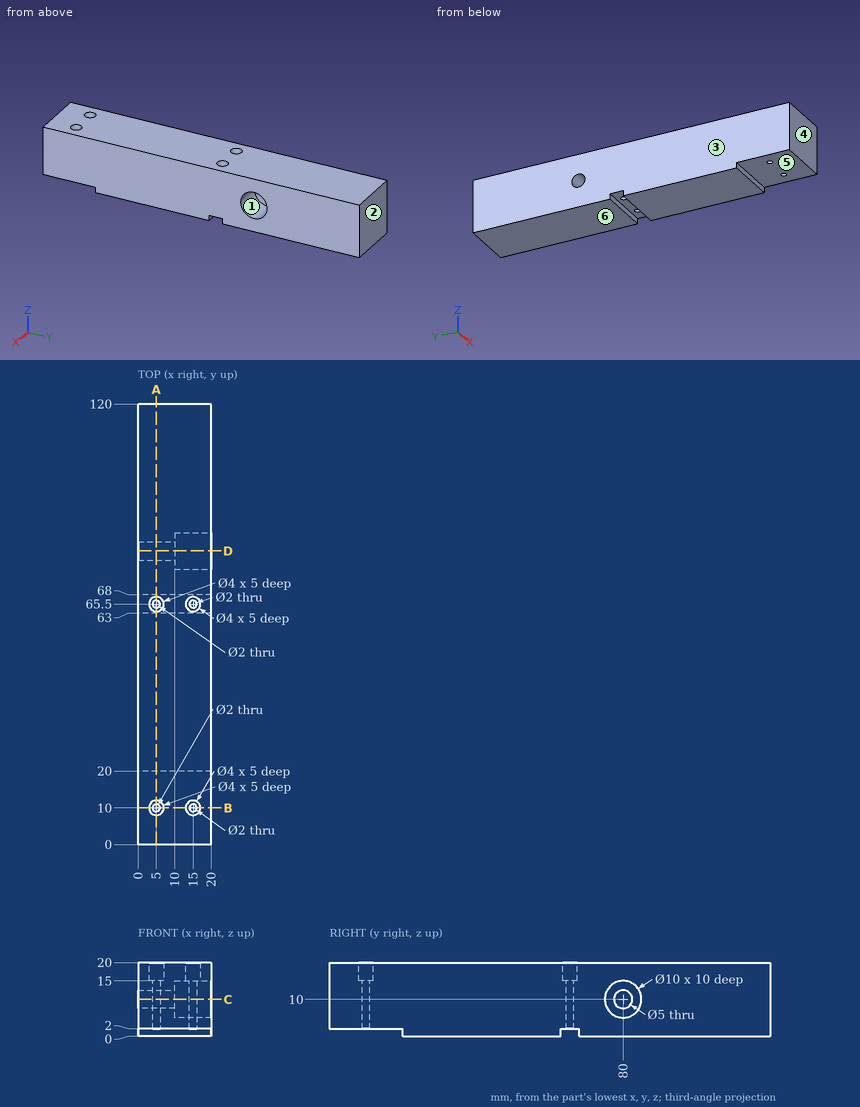
Design review of the part shown in the three views and the two pictorial views. Dimensions are in mm from the part's minimum x, y and z. A direction names the side the tool comes from. Round coordinates to 2 decimals unless told otherwise and drop trailing zeros. Order: outer loops, then holes, each group sorted by start corner. A loop starts at its lowest first (then second) coordinate and runs counter-clockwise, first axis right, second up.
(1) Take a section at A-A, the plane x = 5. State the section outline as (y, z) points.
Working result:
outline: (0, 2) - (9, 2) - (9, 15) - (8, 15) - (8, 20) - (0, 20) - close; (11, 2) - (20, 2) - (20, 0) - (63, 0) - (63, 2) - (64.5, 2) - (64.5, 15) - (63.5, 15) - (63.5, 20) - (12, 20) - (12, 15) - (11, 15) - close; (66.5, 2) - (68, 2) - (68, 0) - (120, 0) - (120, 20) - (67.5, 20) - (67.5, 15) - (66.5, 15) - close; hole circle Ø5 at (80, 10)
(2) Take a section at C-C, the plane z = 10. State the section outline as (x, y) points.
Working result:
outline: (0, 0) - (20, 0) - (20, 75) - (10, 75) - (10, 77.5) - (0, 77.5) - close; (0, 82.5) - (10, 82.5) - (10, 85) - (20, 85) - (20, 120) - (0, 120) - close; hole circle Ø2 at (5, 10); hole circle Ø2 at (5, 65.5); hole circle Ø2 at (15, 10); hole circle Ø2 at (15, 65.5)
(3) Wall thickness on L1, parallel to X at y = 65.5, z = 5.25; L2, parallel to Y at x = 15, z = 10.25; L3, parallel to Y at x = 5, z = 6.75: over which ranges is each line inside the solid? List them lowest first.
Working result:
L1: x = 0 to 4, 6 to 14, 16 to 20
L2: y = 0 to 9, 11 to 64.5, 66.5 to 75.01, 84.99 to 120
L3: y = 0 to 9, 11 to 64.5, 66.5 to 120
(4) Take a section at B-B, the plane y = 10. State the section outline as (x, z) points.
Working result:
outline: (0, 2) - (4, 2) - (4, 15) - (3, 15) - (3, 20) - (0, 20) - close; (6, 2) - (14, 2) - (14, 15) - (13, 15) - (13, 20) - (7, 20) - (7, 15) - (6, 15) - close; (16, 2) - (20, 2) - (20, 20) - (17, 20) - (17, 15) - (16, 15) - close
(5) For P1, Ø2.5, axis at x = 15, y = 10, coming from the -Z side; P2, Ø3, axis at x = 5, y = 10, coming from the +Z side; P3, Ø1, axis at x = 7, z = 1, coming from the -Y side, all flat-tipped, find the tip position at first contact; note any pin that passes through.
Working result:
P1: stops at z = 2
P2: stops at z = 15
P3: stops at y = 20
(6) Mouldability with a two-part tool opening along Y and no side actions: class the marked faces 1, 2, 3 and 4 as released by +Y, released by -Y, zero draft, split by the parting line, or undercut.
Working result:
face 1: undercut
face 2: released by +Y
face 3: zero draft
face 4: released by -Y
(7) Take a section at D-D, the plane y = 80. State the section outline as (x, z) points, plus the area to 3 significant figures.
Working result:
outline: (0, 0) - (20, 0) - (20, 5) - (10, 5) - (10, 7.5) - (0, 7.5) - close; (0, 12.5) - (10, 12.5) - (10, 15) - (20, 15) - (20, 20) - (0, 20) - close
area: 250 mm2
(8) Tool access review of the marked faces 5 and 6: name each direction out of +Z, -Z, +X, -X, +Y, -Y from which nothing blocks a thin tool from reaching the whole face with its end or side.
Working result:
face 5: -Z, +X, -X, -Y
face 6: -Z, +X, -X, +Y, -Y
